```python
from build123d import *

# Parameters (mm, degrees)
F2_SIZE2 = 0.81
F2_SIZE  = 0.81
F3_R     = 0.5


with BuildPart() as f1:
    # F0 (on Front) → F1 (revolve)
    with BuildSketch(Plane.XZ):
        Polygon((0, 6.8), (0, 0), (45, 0), (45, 4.7), (2.1, 4.7), (2.1, 6.8), align=None)
    revolve(axis=Axis((22.5, 0, 0), (1, 0, 0)))

    # F2
    f2_edges = [f1.edges().sort_by_distance(p)[0] for p in [
        (45, 0, -4.7),
    ]]
    chamfer(f2_edges, length=F2_SIZE, length2=F2_SIZE2)

    # F3
    f3_edges = [f1.edges().sort_by_distance(p)[0] for p in [
        (2.1, 0, -6.8),
        (0, 0, -6.8),
        (1.05, 0, 6.8),
    ]]
    fillet(f3_edges, radius=F3_R)


solid = f1.part
```
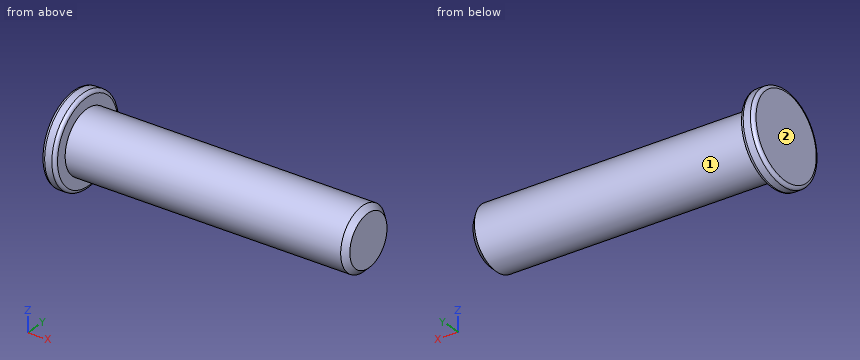
CAD build for the part. Positions are in the model's coordinates, mm. Face numbers are marked on the shaded views. A direction names the side the tool comes from. Coordinates: 2 decimals unless noted, no trailing zeros. Order: outer loops, then holes, each group sorted by start corner. A loop starts at its lowest first (then second) coordinate and runs counter-clockwise, first axis right, second up. Notation, with made-up numbers: (38.25, 67) - (95.25, 67) arc R27 ccw to (95.25, 88) - close; hole circle Ø3 at (14.25, -1.75). An arc over 180 degrees is marked (long way). Answer in a Markdown table with one row per item.
1. 3-axis set-ups, long thin cutter, end or side, ignore diameter. For the marked faces 1 and 2: which of +Z, -Z, +X, -X, +Y, -Y reach the whole face in a straight line?
Answer:
| item | result |
|---|---|
| face 1 | +X |
| face 2 | +Z, -Z, -X, +Y, -Y |
2. Slice it at A-A, the plane y = 0. List the corners of the cut face in (x, z), then the cut area to 3 significant figures.
Answer:
| item | result |
|---|---|
| outline | (0, -6.3) arc R0.5 ccw to (0.5, -6.8) - (1.6, -6.8) arc R0.5 ccw to (2.1, -6.3) - (2.1, -4.7) - (44.19, -4.7) - (45, -3.89) - (45, 3.89) - (44.19, 4.7) - (2.1, 4.7) - (2.1, 6.3) arc R0.5 ccw to (1.6, 6.8) - (0.5, 6.8) arc R0.5 ccw to (0, 6.3) - close |
| area | 431 mm² |
3. Drill centre lines: L1, parallel to Z at x = 42, y = 0; L2, parallel to X at y = -2.5, z = 5.75. Where is each one in solid material? Low to high. Write a range as from..to.
Answer:
| item | result |
|---|---|
| L1 | -4.7..4.7 |
| L2 | 0..2.1 |
4. Flat gauge pins, fed straight in: P1, Ø2, axis at y = 1.5, z = -5, coming from the +X side; P2, Ø8, axis at x = 35, y = -1, coming from the -Z side; P3, Ø3, axis at x = 15.5, y = -2.5, coming from the +Z side. Where does each tip first touch, or does it go through?
Answer:
| item | result |
|---|---|
| P1 | x = 44.67 |
| P2 | z = -4.7 |
| P3 | z = 4.59 |
5. Slice it at C-C, the plane x = 18. List the corners of the cut face in (y, z), then the cut area to 3 significant figures.
Answer:
| item | result |
|---|---|
| outline | circle Ø9.4 at (0, 0) |
| area | 69.4 mm² |
